Can you work these out from the model? Positions are in its coordinate system, mm. A direction names the side the tool comes from. Round coordinates to 2 decimals unless told otherwise and drop trailing zeros. Order: outer loops, then holes, each group sorted by start corner. A loop starts at its lowest first (then second) coordinate and runs counter-clockwise, first axis right, second up.
Q1. Will these pins go through, and if not, where does the flat tip stop? P1, Ø1.5, axis at x = -27, z = 1, coming from the +Y side; P2, Ø3.5, axis at x = 28.125, y = 14.5, coming from the -Z side; P3, Ø2.5, axis at x = -14.68, y = 20.25, coming from the +Z side (1 decimal).
Q2. If we section it at A-A (y = 14.5): Please give me the cut outline in (x, z) (3 decimals), plus the area to 3 significant figures.
Q3. We'd pull the mould along Y, two halves only. Please class faces 1 (the face through (38.125, 1, 10)), 2 (the face through (-35.625, 12, 31)), 3 (the face through (-1, 1.5, 0)): pulls with the +Y half, pulls with the -Y half, needs draft (parallel to the pull), parting line crosses it, or undercut.
Q4. If I drill on line 1 (Y direction, x = 24, z = -16); line 2 (Z direction, x = -25.5, y = 18); line 3 (Y direction, x = 28.5, z = 29.5), over which ranges is the centre line in solid material (lowest first)?
Q5. If we section it at D-D (z = 8): Please give me the cut outline in (x, y) (3 decimals).
Q6. For faces 4 (the face through (-1, 13, 29.2)), 5 (the face through (-31.125, 13, 31)), 6 (the face through (-1, 25, 31)), which set-ups out of +Z, -Z, +X, -X, +Y, -Y let a thin tool reach every point of the face, with its end or its side?
Q7. If we section it at C-C (y = 3.25): Please give me the cut outline in (x, z) (3 decimals).
Q8. If we section it at B-B (x = 20): Please give me the cut outline in (y, z).
from build123d import *

# Parameters (mm, degrees)
SKETCH1_W           = 76.25
SKETCH1_H           = 58.4
BOSS_EXTRUDE1_DEPTH = 1.5
SKETCH2_W           = 76.25
SKETCH2_H           = 25
BOSS_EXTRUDE2_DEPTH = 3
SKETCH3_R           = 1.5
CUT_EXTRUDE1_DEPTH  = 77.475326904


with BuildPart() as part:
    # Sketch1 → Boss-Extrude1 (new body)
    with BuildSketch(Plane(origin=(0, 0, 0), x_dir=(1, 0, 0), z_dir=(0, 1, 0))):
        Rectangle(SKETCH1_W, SKETCH1_H)
    extrude(amount=BOSS_EXTRUDE1_DEPTH)

    # Sketch2 → Boss-Extrude2 (add)
    with BuildSketch(Plane.XY.offset(29.2)):
        with Locations((0, 12.5)):
            Rectangle(SKETCH2_W, SKETCH2_H)
    extrude(amount=BOSS_EXTRUDE2_DEPTH)

    # Sketch3 → Cut-Extrude1 (cut, through all)
    with BuildSketch(Plane.XY.offset(32.2)):
        with Locations((-28.125, 14.5)):
            Circle(SKETCH3_R)
        with Locations((-14.678089157, 20.247551858)):
            Circle(SKETCH3_R)
        with BuildLine():
            Line((-31.125, 18.55), (-31.125, 6.45))
            ThreePointArc((-31.125, 6.45), (-33.375, 4.2), (-35.625, 6.45))
            Line((-35.625, 6.45), (-35.625, 18.55))
            ThreePointArc((-35.625, 18.55), (-33.375, 20.8), (-31.125, 18.55))
        make_face()
    cut_extrude1 = extrude(amount=-CUT_EXTRUDE1_DEPTH, mode=Mode.SUBTRACT)

    # Mirror1: Cut-Extrude1 across plane
    add(cut_extrude1.mirror(Plane(origin=(0, 0, 0), x_dir=(0, 0, 1), z_dir=(1, 0, 0))), mode=Mode.SUBTRACT)


solid = part.part
Solution:
1. P1: stops at y = 1.5
1. P2: stops at z = 29.2
1. P3: passes through
2. outline: (-38.125, 29.2) - (-35.625, 29.2) - (-35.625, 32.2) - (-38.125, 32.2) - close; (-31.125, 29.2) - (-29.625, 29.2) - (-29.625, 32.2) - (-31.125, 32.2) - close; (-26.625, 29.2) - (26.625, 29.2) - (26.625, 32.2) - (-26.625, 32.2) - close; (29.625, 29.2) - (31.125, 29.2) - (31.125, 32.2) - (29.625, 32.2) - close; (35.625, 29.2) - (38.125, 29.2) - (38.125, 32.2) - (35.625, 32.2) - close
2. area: 184 mm2
3. face 1: needs draft
3. face 2: undercut
3. face 3: pulls with the +Y half
4. line 1: y = 0 to 1.5
4. line 2: z = 29.2 to 32.2
4. line 3: y = 0 to 13.05, 15.95 to 25
5. outline: (-38.125, 0) - (38.125, 0) - (38.125, 1.5) - (-38.125, 1.5) - close
6. face 4: -Z, +X, -X, +Y
6. face 5: +Z, -Z
6. face 6: +Z, -Z, +X, -X, +Y
7. outline: (-38.125, 29.2) - (38.125, 29.2) - (38.125, 32.2) - (-38.125, 32.2) - close
8. outline: (0, -29.2) - (1.5, -29.2) - (1.5, 29.2) - (25, 29.2) - (25, 32.2) - (0, 32.2) - close
